```python
from build123d import *

# Parameters (mm, degrees)
BOSS_EXTRUDE1_DEPTH  = 19.05
M5_CLEARANCE_HOLE1_D = 5.3
FILLET1_R            = 8


with BuildPart() as part:
    # Sketch1 → Boss-Extrude1 (new, symmetric)
    with BuildSketch(Plane.XY):
        Polygon((0, 0), (34.5, 0), (34.5, 8), (8, 8), align=None)
    extrude(amount=BOSS_EXTRUDE1_DEPTH, both=True)

    # M5 Clearance Hole1 (through all)
    with Locations(Plane(origin=(0, 8, 0), x_dir=(1, 0, 0), z_dir=(0, 1, 0))):
        with Locations((25.4, 12.7), (25.4, -12.7)):
            Hole(M5_CLEARANCE_HOLE1_D / 2)

    # Mirror1: part across plane


with BuildPart() as part_1:
    add(part.part)
    add(part.part.mirror(Plane(origin=(0, 0, 19.05), x_dir=(0, 0, 1), z_dir=(0.7071067811865475, -0.7071067811865478, 0))))

    # Fillet1
    fillet1_edges = [part_1.edges().sort_by_distance(p)[0] for p in [
        (8, 8, 0),
    ]]
    fillet(fillet1_edges, radius=FILLET1_R)


solid = part_1.part
```
Check sheet for the modelled part. Datum: model origin and axes. Units: mm. A direction names the side the tool comes from. Round coordinates to 2 decimals unless told otherwise and drop trailing zeros. Loops run counter-clockwise (first coordinate to the right, second up) from the corner with the lowest first, then second, coordinate; pieces in that order, holes last. Notation, with made-up numbers: (11.5, -11) - (58.5, -11) arc R25 ccw to (58.5, 24) - close; hole circle Ø1 at (-26.5, -23). An arc over 180 degrees is marked (long way). Write item = value, one per line. Start each with the question number.
Q1. Section check B-B (y = 25.4). Record the boundary of the cut face in (x, z), plus the area to 3 significant figures.
Q2. Thickness scan on L1, parallel to Z at x = 25.4, y = 4; L2, parallel to X at y = 5, z = -12.5; L3, parallel to Y at x = 3.5, z = -12.7. Record the ranges inside material, lowest first.
Q3. Section check A-A (z = -12.7). Record the boundary of the cut face in (x, y).
Q4. Section check D-D (y = 5.5). Record the boundary of the cut face in (x, z), plus the area to 3 significant figures.
Q5. Release check for a two-part mould opening along Z. For faces 3 (the face through (25, 8, 0)), 4 (the face through (10, 9, -19.05)), 5 (the face through (22.95, 3.94, -11.69)) record: pulls with the +Z half, pulls with the -Z half, needs draft (parallel to the pull), parting line crosses it, or undercut.
Q6. Depth check by flat-ended pin: P1, Ø8.5, axis at y = 25.4, z = 12.7, coming from the +X side; P2, Ø5.5, axis at x = 22.5, z = -6, coming from the +Y side. Enter the tip coordinate at first touch or a pass-through.
Q7. Access from +Z, -Z, +X, -X, +Y, -Y to the whole of each face (thin tool, end or side, straight path). Record for faces 1 (the face through (4, 34.5, 0)), 2 (the face through (8, 25, 0)).
Derived:
q1.outline = (0, -19.05) - (8, -19.05) - (8, -15.35) - (0, -15.35) - close; (0, -10.05) - (8, -10.05) - (8, 10.05) - (0, 10.05) - close; (0, 15.35) - (8, 15.35) - (8, 19.05) - (0, 19.05) - close
q1.area = 220 mm^2
q2.L1 = -19.05 to -15.35, -10.05 to 10.05, 15.35 to 19.05
q2.L2 = 0 to 22.76, 28.04 to 34.5
q2.L3 = 0 to 22.75, 28.05 to 34.5
q3.outline = (0, 0) - (22.75, 0) - (22.75, 8) - (16, 8) arc R8 cw to (8, 16) - (8, 22.75) - (0, 22.75) - close; (0, 28.05) - (8, 28.05) - (8, 34.5) - (0, 34.5) - close; (28.05, 0) - (34.5, 0) - (34.5, 8) - (28.05, 8) - close
q4.outline = (0, -19.05) - (34.5, -19.05) - (34.5, 19.05) - (0, 19.05) - close; hole circle Ø5.3 at (25.4, -12.7); hole circle Ø5.3 at (25.4, 12.7)
q4.area = 1,270 mm^2
q5.face_3 = needs draft
q5.face_4 = pulls with the -Z half
q5.face_5 = undercut
q6.P1 = 8
q6.P2 = 8
q7.face_1 = +Z, -Z, +X, -X, +Y
q7.face_2 = +Z, -Z, +X, +Y
